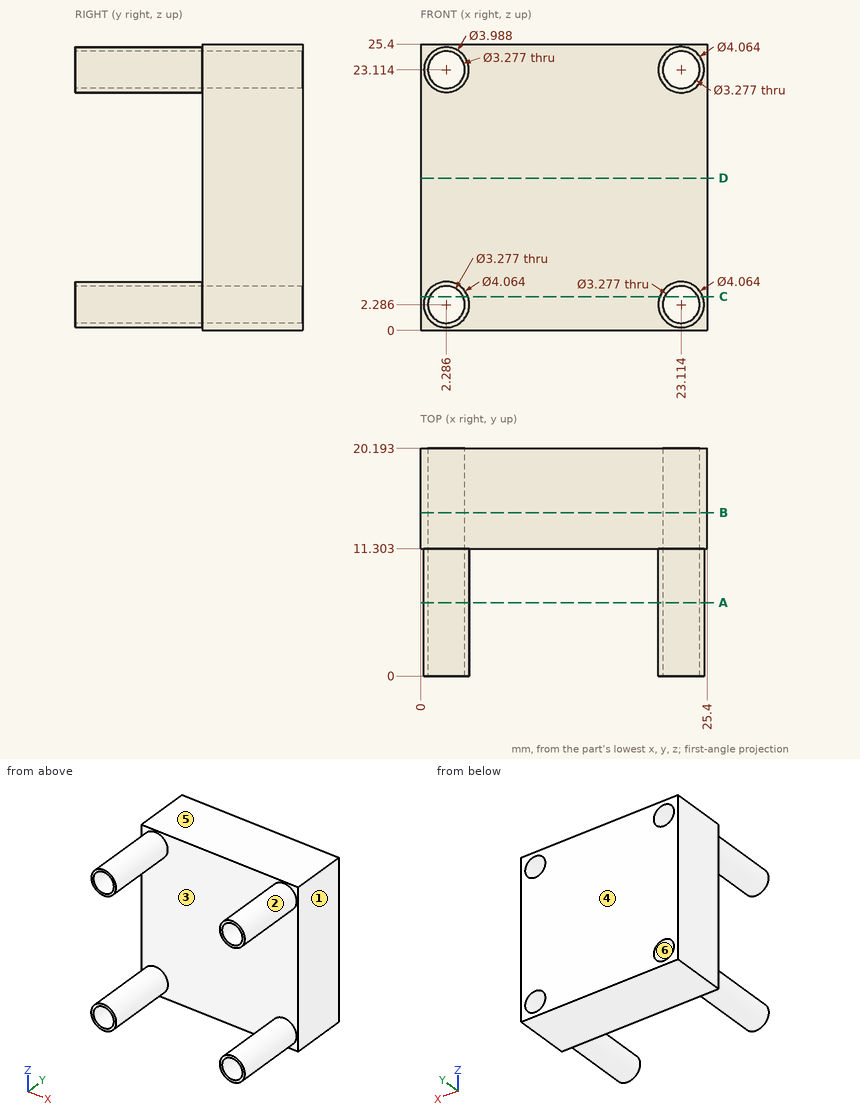
Can you work these out from the drawing? Everything is in mm from the part's minimum corner. A direction names the side the tool comes from. Round coordinates to 2 decimals unless told otherwise and drop trailing zeros. Write each loop counter-clockwise with the first axis right and the second up, starting at its lowest first coordinate (ties: lowest second). Pieces come first, ordered by that corner, then holes. Notation, with made-up numbers: (87, 45) - (93, 45) arc R25 cw to (93, 59) - close; hole circle Ø5 at (-38.5, 34.25). An arc over 180 degrees is marked (long way). Write each question's results on one line, items separated by ' | '. Start each with the question number.
1) Suppose I cut it at B-B (y = 14.5). List the corners of the cut face in (x, z) for me (1 decimal).
2) We'd pull the mould along Z, two halves only. Please class the marked faces 3, 4, 5 and 6: released by +Z, released by -Z, zero draft, split by the parting line, or undercut.
3) Which directions (+Z, -Z, +X, -X, +Y, -Y) give clear straight access to the entire face, cutting with the end or side of a thin tool? Please do the marked faces 1 and 2.
4) Please list where these lines run through material, in increasing order: line 1 (X direction, y = 7.5, z = 21.75) (1 decimal); line 2 (X direction, y = 12, z = 21.75) (1 decimal); line 3 (X direction, y = 1.25, z = 22.75) (1 decimal).
5) Suppose I cut it at C-C (z = 3). List the corners of the cut face in (x, y) for me.
6) Suppose I cut it at A-A (y = 6.5). List the corners of the cut face in (x, z) for me (1 decimal).
7) Suppose I cut it at D-D (z = 13.5). List the corners of the cut face in (x, y) for me.
8) For pin 1 Ø2 at (x, z) = (16.5, 4) entering from -Y, with a flat end and sliding along its axis, tell me the tip position at first contact or that it passes through.
Here are the results:
1) outline: (0, 0) - (25.4, 0) - (25.4, 25.4) - (0, 25.4) - close; hole circle Ø3.3 at (2.3, 2.3); hole circle Ø3.3 at (2.3, 23.1); hole circle Ø3.3 at (23.1, 2.3); hole circle Ø3.3 at (23.1, 23.1)
2) face 3: undercut | face 4: zero draft | face 5: released by +Z | face 6: undercut
3) face 1: +Z, -Z, +X, +Y, -Y | face 2: -Y
4) line 1: x = 0.8 to 1.4, 3.2 to 3.7, 21.6 to 22.2, 24 to 24.6 | line 2: x = 0 to 1.4, 3.2 to 22.2, 24 to 25.4 | line 3: x = 0.3 to 0.7, 3.9 to 4.2, 21.1 to 21.5, 24.7 to 25.1
5) outline: (0, 11.3) - (0.38, 11.3) - (0.38, 0) - (0.81, 0) - (0.81, 20.19) - (0, 20.19) - close; (3.76, 0) - (4.19, 0) - (4.19, 11.3) - (21.21, 11.3) - (21.21, 0) - (21.64, 0) - (21.64, 20.19) - (3.76, 20.19) - close; (24.59, 0) - (25.02, 0) - (25.02, 11.3) - (25.4, 11.3) - (25.4, 20.19) - (24.59, 20.19) - close
6) outline: circle Ø4.1 at (2.3, 2.3); circle Ø4 at (2.3, 23.1); circle Ø4.1 at (23.1, 2.3); circle Ø4.1 at (23.1, 23.1); hole circle Ø3.3 at (2.3, 2.3); hole circle Ø3.3 at (2.3, 23.1); hole circle Ø3.3 at (23.1, 2.3); hole circle Ø3.3 at (23.1, 23.1)
7) outline: (0, 11.3) - (25.4, 11.3) - (25.4, 20.19) - (0, 20.19) - close
8) pin 1: stops at y = 11.3
